Autodesk Inventor part; units mm, degrees
ref_plane "YZ Plane" through (0, 0, 0) normal (1, 0, 0) x (0, 1, 0)
ref_plane "XZ Plane" through (0, 0, 0) normal (0, 1, 0) x (-1, 0, 0)
ref_plane "XY Plane" through (0, 0, 0) normal (0, 0, 1) x (1, 0, 0)
sketch "Sketch1" plane through (0, 0, 0) normal (0, 1, 0) x (-1, 0, 0)
  line L0 (0, 0) -> (0, -25.4)
  line L1 (0, 0) -> (0, 3.302)
  line L2 (0, 3.302) -> (25.4, 3.302)
  line L3 (25.4, 3.302) -> (25.4, 0)
  line L4 (0, -25.4) -> (3.302, -25.4)
  line L5 (3.302, -25.4) -> (3.302, 0)
  line L6 (3.302, 0) -> (25.4, 0)
  dimension "d0" = 25.4
  dimension "d1" = 3.302
  dimension "d2" = 25.4
  dimension "d3" = 3.302
extrude "Extrusion1" add sketch "Sketch1" along normal blind 88.9
properties part number "Winch Upright Bracket"
Could you check a few things on this model? Use its own coordinates, in mm. A direction names the side the tool comes from. Coordinates: 2 decimals unless noted, no trailing zeros. Order: outer loops, then holes, each group sorted by start corner. A loop starts at its lowest first (then second) coordinate and runs counter-clockwise, first axis right, second up.
Q1. Please list where these lines run through material, in increasing order: L1, parallel to X at y = 65.5, z = -19.75; L2, parallel to Z at x = -18.5, y = 63.
Q2. Suppose I cut it at A-A on y = 69. Please give me the cut outline in (x, z).
Q3. Will these pins go through, and if not, where does the flat tip stop? pin 1 (7.5 mm diameter, centred on y = 43.5, z = -12, fed in from -X); pin 2 (2 mm diameter, centred on x = -10.5, y = 78, fed in from -Z).
Q4. Suppose I cut it at C-C on x = -21. Please give me the cut outline in (y, z), and give its area (3 significant figures).
Q5. Suppose I cut it at B-B on z = -10.25. Please give me the cut outline in (x, y), and give its area (3 significant figures).
Q6. Which directions (+Z, -Z, +X, -X, +Y, -Y) give clear straight access to the entire face, cutting with the end or side of a thin tool? Please do faces 1 (the flat face through (-3, 0, -7)), 2 (the flat face through (-14, 44, 0)).
Answer:
1. L1: x = -3.3 to 0
1. L2: z = 0 to 3.3
2. outline: (-25.4, 0) - (-3.3, 0) - (-3.3, -25.4) - (0, -25.4) - (0, 3.3) - (-25.4, 3.3) - close
3. pin 1: stops at x = -3.3
3. pin 2: stops at z = 0
4. outline: (0, 0) - (88.9, 0) - (88.9, 3.3) - (0, 3.3) - close
4. area: 294 mm2
5. outline: (-3.3, 0) - (0, 0) - (0, 88.9) - (-3.3, 88.9) - close
5. area: 294 mm2
6. face 1: +Z, -Z, +X, -X, -Y
6. face 2: -Z, -X, +Y, -Y
